Source: CAD feature listing. Evaluate the final solid. Frame: model axes, mm. Round coordinates to 2 decimals unless told otherwise and drop trailing zeros. Answer as CSV lines item,"result". Start each with the question number.
Item 1: Pull-direction query (Y, two-part tool) for faces 1 (the face through (46.62, -40.18, 1.57)), 2 (the face through (-46.073, -40.641, 1.565)), 3 (the face through (-53.1, -1, 2)), 4 (the face through (51, 47.5, 2)); classes: +Y half, -Y half, draft (parallel to the pull), parting line (faces both ways), or undercut.
Item 2: Line query: line 1 (Y direction, x = 48.1, z = 1.9). Output: solid intervals per line, ascending. Write a range as [from, to].
Item 3: First-contact query: P1, Ø5, axis at x = -48.1, y = -42.5, coming from the +Z side. Flat tip, straight axial feed; report the tip coordinate or a pass-through.
from build123d import *

# Parameters (mm, degrees)
SKETCH1_W           = 106.2
SKETCH1_H           = 95
BOSS_EXTRUDE1_DEPTH = 3.175
CUT_EXTRUDE1_REACH  = 73.316
SKETCH2_R           = 2.75


with BuildPart() as part:
    # Sketch1 → Boss-Extrude1 (new body)
    with BuildSketch(Plane.XY):
        Rectangle(SKETCH1_W, SKETCH1_H)
    extrude(amount=BOSS_EXTRUDE1_DEPTH)

    # Sketch2 → Cut-Extrude1 (cut, up to next)
    with BuildSketch(Plane(origin=(0, 0, 0), x_dir=(-1, 0, 0), z_dir=(0, 0, -1)), mode=Mode.PRIVATE) as cut_extrude1_sk1:
        with Locations((-48.1, 50.21)):
            Circle(SKETCH2_R)
    cut_extrude1_tool1 = extrude(cut_extrude1_sk1.sketch, amount=-CUT_EXTRUDE1_REACH, mode=Mode.PRIVATE) & part.part
    # Sketch2 → Cut-Extrude1 (cut, up to next)
    with BuildSketch(Plane(origin=(0, 0, 0), x_dir=(-1, 0, 0), z_dir=(0, 0, -1)), mode=Mode.PRIVATE) as cut_extrude1_sk2:
        with Locations((-48.1, -42.5)):
            Circle(SKETCH2_R)
    cut_extrude1_tool2 = extrude(cut_extrude1_sk2.sketch, amount=-CUT_EXTRUDE1_REACH, mode=Mode.PRIVATE) & part.part
    # Sketch2 → Cut-Extrude1 (cut, up to next)
    with BuildSketch(Plane(origin=(0, 0, 0), x_dir=(-1, 0, 0), z_dir=(0, 0, -1)), mode=Mode.PRIVATE) as cut_extrude1_sk3:
        with Locations((48.1, -42.5)):
            Circle(SKETCH2_R)
    cut_extrude1_tool3 = extrude(cut_extrude1_sk3.sketch, amount=-CUT_EXTRUDE1_REACH, mode=Mode.PRIVATE) & part.part
    # Sketch2 → Cut-Extrude1 (cut, up to next)
    with BuildSketch(Plane(origin=(0, 0, 0), x_dir=(-1, 0, 0), z_dir=(0, 0, -1)), mode=Mode.PRIVATE) as cut_extrude1_sk4:
        with Locations((48.1, 50.21)):
            Circle(SKETCH2_R)
    cut_extrude1_tool4 = extrude(cut_extrude1_sk4.sketch, amount=-CUT_EXTRUDE1_REACH, mode=Mode.PRIVATE) & part.part
    add(cut_extrude1_tool1.solids().sort_by_distance((48.1, 50.21, 0))[0], mode=Mode.SUBTRACT)
    add(cut_extrude1_tool2.solids().sort_by_distance((48.1, -42.5, 0))[0], mode=Mode.SUBTRACT)
    add(cut_extrude1_tool3.solids().sort_by_distance((-48.1, -42.5, 0))[0], mode=Mode.SUBTRACT)
    add(cut_extrude1_tool4.solids().sort_by_distance((-48.1, 50.21, 0))[0], mode=Mode.SUBTRACT)


solid = part.part
Results:
1,face 1,"undercut"
1,face 2,"undercut"
1,face 3,"draft"
1,face 4,"+Y half"
2,line 1,"[-47.5, -45.25], [-39.75, 47.46]"
3,P1,"through"
